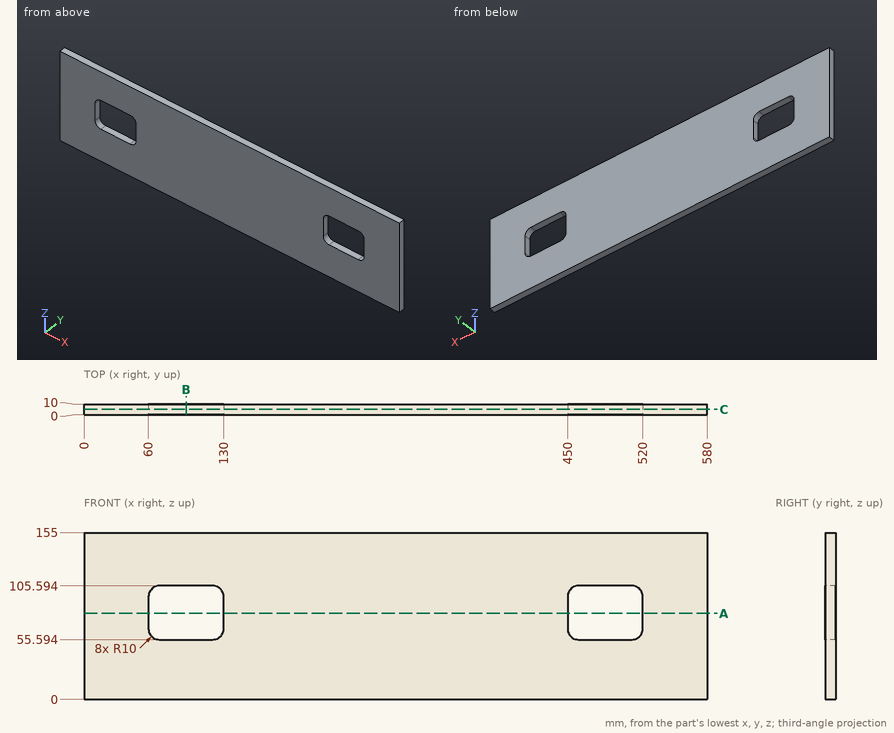
For this review, use the dimensioned drawing (mm, ordinates from the lowest corner) and the shaded views. Coordinates: 2 decimals unless noted, no trailing zeros. Write each loop counter-clockwise with the first axis right and the second up, starting at its lowest first coordinate (ties: lowest second). Pieces come first, ordered by that corner, then holes. Notation, with made-up numbers: (-40, 2) - (-13, 2) arc R28 ccw to (-13, 35) - close; hole circle Ø9 at (76, -34.5). An arc over 180 degrees is marked (long way). Answer as a JSON object with one key per item and string values. Group by question number.
1. Add section C-C (y = 5). Give the boundary of the cut face in (x, z), plus the area to 3 significant figures.
2. Add section A-A (z = 80). Give the boundary of the cut face in (x, y), plus the area to 3 significant figures.
3. Add section B-B (x = 95). Give the boundary of the cut face in (y, z), plus the area to 3 significant figures.
4. To check wall thickness, follow probe 1 along X at (y, z) = (6.25, 84); probe 2 along X at (y, z) = (0.75, 57); probe 3 along Z at (x, y) = (119.5, 7). State the ranges of each line that lie inside material, in increasing order.
Findings:
{
 "1": {"outline": "(0, 0) - (580, 0) - (580, 155) - (0, 155) - close; hole (60, 65.59) arc R10 ccw to (70, 55.59) - (120, 55.59) arc R10 ccw to (130, 65.59) - (130, 95.59) arc R10 ccw to (120, 105.59) - (70, 105.59) arc R10 ccw to (60, 95.59) - close; hole (450, 65.59) arc R10 ccw to (460, 55.59) - (510, 55.59) arc R10 ccw to (520, 65.59) - (520, 95.59) arc R10 ccw to (510, 105.59) - (460, 105.59) arc R10 ccw to (450, 95.59) - close", "area": "83,100 mm²"},
 "2": {"outline": "(0, 0) - (60, 0) - (60, 10) - (0, 10) - close; (130, 0) - (450, 0) - (450, 10) - (130, 10) - close; (520, 0) - (580, 0) - (580, 10) - (520, 10) - close", "area": "4,400 mm²"},
 "3": {"outline": "(0, 0) - (10, 0) - (10, 55.59) - (0, 55.59) - close; (0, 105.59) - (10, 105.59) - (10, 155) - (0, 155) - close", "area": "1,050 mm²"},
 "4": {"probe 1": "0 to 60, 130 to 450, 520 to 580", "probe 2": "0 to 64.89, 125.11 to 454.89, 515.11 to 580", "probe 3": "0 to 55.59, 105.59 to 155"}
}
